```python
from build123d import *

# Parameters (mm, degrees)
SKETCH1_R           = 5
BOSS_EXTRUDE1_DEPTH = 30
SKETCH2_R           = 2
CUT_EXTRUDE1_DEPTH  = 31
CUT_EXTRUDE2_DEPTH  = 3
LPATTERN1_COUNT     = 2
LPATTERN1_PITCH     = 27


with BuildPart() as part:
    # Sketch1 → Boss-Extrude1 (new body)
    with BuildSketch(Plane(origin=(0, 0, 0), x_dir=(1, 0, 0), z_dir=(0, 1, 0))):
        Circle(SKETCH1_R)
    extrude(amount=BOSS_EXTRUDE1_DEPTH)

    # Sketch2 → Cut-Extrude1 (cut, through all)
    with BuildSketch(Plane(origin=(0, 30, 0), x_dir=(1, 0, 0), z_dir=(0, 1, 0))):
        Circle(SKETCH2_R)
    extrude(amount=-CUT_EXTRUDE1_DEPTH, mode=Mode.SUBTRACT)

    # Sketch3 → Cut-Extrude2 (cut)
    with BuildSketch(Plane(origin=(0, 30, 0), x_dir=(1, 0, 0), z_dir=(0, 1, 0))):
        Polygon((1.599030575, -2.74343481), (3.175399526, 0.013083694), (1.576368951, 2.756518504), (-1.599030575, 2.74343481), (-3.175399526, -0.013083694), (-1.576368951, -2.756518504), align=None)
    cut_extrude2 = extrude(amount=-CUT_EXTRUDE2_DEPTH, mode=Mode.SUBTRACT)

    # LPattern1: Cut-Extrude2 ×2
    with Locations(*[(0, -i * LPATTERN1_PITCH, 0) for i in range(1, LPATTERN1_COUNT)]):
        add(cut_extrude2, mode=Mode.SUBTRACT)


solid = part.part
```
Verification items for the finished model (mm, model axes). A direction names the side the tool comes from. Give positions to 0.01 mm unless a question says otherwise; leave off trailing zeros. Order: outer loops, then holes, each group sorted by start corner. A loop starts at its lowest first (then second) coordinate and runs counter-clockwise, first axis right, second up. Notation, with made-up numbers: M 26.25,47 L 36.25,47 A16 ccw 36.25,66 Z; hole C 47.5,-29 d8. An arc over 180 degrees is marked long. Return JSON: item names as keys, results as strings. Group by question number.
1) Section check C-C on x = 0. Record the cut outline in (y, z), and give its area (3 significant figures).
2) Mould release check, pull along X, two halves, no side actions. Record for faces 4 (the face through (2.2, 30, 2.2)), 5 (the face through (2, 27, -1)), 6 (the face through (-2.387, 1.521, 1.366)), 7 (the face through (-1.08, 14.79, 4.88)): pulls with the +X half, pulls with the -X half, needs draft (parallel to the pull), parting line crosses it, or undercut.
3) Go/stop test with flat-tipped pins: pin 1 Ø2 at (y, z) = (12, -3.5) entering from +X; pin 2 Ø3 at (x, z) = (-0.5, -0.5) entering from +Y; pin 3 Ø3 at (x, z) = (-0.5, -0.5) entering from -Y. Record where each tip stops, or that it passes through.
4) Section check D-D on z = -3.25. Record the cut outline in (x, y).
5) Section check B-B on z = -1. Record the cut outline in (x, y), and give its area (3 significant figures).
6) Scan lines: line 1 (X direction, y = 12.75, z = 0); line 2 (Y direction, x = -2, z = 1.75). Record each from-to range of solid material in increasing order.
7) Access from +Z, -Z, +X, -X, +Y, -Y to the whole of each face (thin tool, end or side, straight path). Record for faces 1 (the face through (0, 15, 2)), 2 (the face through (-2.387, 28.521, 1.366)), 3 (the face through (2.38, 1.52, 1.38)).
8) Section check A-A on y = 28. Record the cut outline in (x, z), and give its area (3 significant figures).
Answer block:
{
 "1": {"outline": "M 0,-5 L 30,-5 L 30,-2.75 L 27,-2.75 L 27,-2 L 3,-2 L 3,-2.75 L 0,-2.75 Z; M 0,2.75 L 3,2.75 L 3,2 L 27,2 L 27,2.75 L 30,2.75 L 30,5 L 0,5 Z", "area": "171 mm^2"},
 "2": {"face 4": "needs draft", "face 5": "undercut", "face 6": "undercut", "face 7": "parting line crosses it"},
 "3": {"pin 1": "stops at x = 4.33", "pin 2": "stops at y = 27", "pin 3": "stops at y = 3"},
 "4": {"outline": "M -3.8,0 L 3.8,0 L 3.8,30 L -3.8,30 Z"},
 "5": {"outline": "M -4.9,0 L -2.6,0 L -2.6,3 L -1.73,3 L -1.73,27 L -2.6,27 L -2.6,30 L -4.9,30 Z; M 1.73,3 L 2.6,3 L 2.6,0 L 4.9,0 L 4.9,30 L 2.6,30 L 2.6,27 L 1.73,27 Z", "area": "180 mm^2"},
 "6": {"line 1": "x = -5 to -2, 2 to 5", "line 2": "y = 3 to 27"},
 "7": {"face 1": "+Y, -Y", "face 2": "+Y", "face 3": "-Y"},
 "8": {"outline": "C 0,0 d10; hole M -3.18,0.01 L -1.6,-2.74 L 1.58,-2.76 L 3.18,-0.01 L 1.6,2.74 L -1.58,2.76 Z", "area": "52.3 mm^2"}
}
